Source: CAD feature listing. Evaluate the final solid. Frame: model axes, mm. Face numbers are marked on the shaded views. A direction names the side the tool comes from. Give positions to 0.01 mm unless a question says otherwise; leave off trailing zeros. Order: outer loops, then holes, each group sorted by start corner. A loop starts at its lowest first (then second) coordinate and runs counter-clockwise, first axis right, second up. Notation, with made-up numbers: (-23, 73.25) -> (-18, 73.25) arc R14 cw to (-18, 99.25) -> close; hole circle Ø11 at (-29, 5.5). An arc over 180 degrees is marked (long way). Answer in a Markdown table with one row per item.
```python
from build123d import *

# Parameters (mm, degrees)
SKETCH1_R           = 2
BOSS_EXTRUDE1_DEPTH = 3
SKETCH2_R           = 7
BOSS_EXTRUDE2_DEPTH = 9.35
SKETCH3_R           = 7.5
BOSS_EXTRUDE3_DEPTH = 0.5
SKETCH4_W           = 3
SKETCH4_H           = 9
BOSS_EXTRUDE4_DEPTH = 24.5
SKETCH5_R           = 6
BOSS_EXTRUDE5_DEPTH = 9.5
SKETCH8_R           = 5.5
BOSS_EXTRUDE6_DEPTH = 1.65
SKETCH9_R           = 7
BOSS_EXTRUDE7_DEPTH = 2
SKETCH10_R          = 4.5
CUT_EXTRUDE1_DEPTH  = 25
CUT_EXTRUDE2_DEPTH  = 3


with BuildPart() as part:
    # Sketch1 → Boss-Extrude1 (new body)
    with BuildSketch(Plane.XY):
        with BuildLine():
            ThreePointArc((-3.999511648, -14.062500079), (-8.7e-08, -16.5), (3.999511568, -14.062500234))
            Line((3.999511568, -14.062500234), (8.887803753, -4.583333333))
            ThreePointArc((8.887803753, -4.583333333), (10, 0), (8.887803753, 4.583333333))
            Line((8.887803753, 4.583333333), (3.999511579, 14.062500214))
            ThreePointArc((3.999511579, 14.062500214), (-6.7e-08, 16.5), (-3.99951164, 14.062500095))
            Line((-3.99951164, 14.062500095), (-8.887803753, 4.583333333))
            ThreePointArc((-8.887803753, 4.583333333), (-10, 0), (-8.887803753, -4.583333333))
            Line((-8.887803753, -4.583333333), (-3.999511648, -14.062500079))
        make_face()
        with Locations((0, -12)):
            Circle(SKETCH1_R, mode=Mode.SUBTRACT)
        with Locations((0, 12)):
            Circle(SKETCH1_R, mode=Mode.SUBTRACT)
    extrude(amount=BOSS_EXTRUDE1_DEPTH)

    # Sketch2 → Boss-Extrude2 (add)
    with BuildSketch(Plane.XY.offset(3)):
        Circle(SKETCH2_R)
    extrude(amount=BOSS_EXTRUDE2_DEPTH)

    # Sketch3 → Boss-Extrude3 (add)
    with BuildSketch(Plane(origin=(0, 0, 0), x_dir=(-1, 0, 0), z_dir=(0, 0, -1))):
        with Locations(Location((0, 0, 0), (0, 0, 180))):
            Circle(SKETCH3_R)
    extrude(amount=BOSS_EXTRUDE3_DEPTH)

    # Sketch4 → Boss-Extrude4 (add)
    with BuildSketch(Plane(origin=(0, 0, -0.5), x_dir=(-1, 0, 0), z_dir=(0, 0, -1))):
        Rectangle(SKETCH4_W, SKETCH4_H)
    extrude(amount=BOSS_EXTRUDE4_DEPTH)

    # Sketch5 → Boss-Extrude5 (add)
    with BuildSketch(Plane(origin=(0, 0, -0.5), x_dir=(-1, 0, 0), z_dir=(0, 0, -1))):
        Circle(SKETCH5_R)
    extrude(amount=BOSS_EXTRUDE5_DEPTH)

    # Sketch8 → Boss-Extrude6 (add)
    with BuildSketch(Plane.XY.offset(12.35)):
        Circle(SKETCH8_R)
    extrude(amount=BOSS_EXTRUDE6_DEPTH)

    # Sketch9 → Boss-Extrude7 (add)
    with BuildSketch(Plane.XY.offset(14)):
        Circle(SKETCH9_R)
    extrude(amount=BOSS_EXTRUDE7_DEPTH)

    # Sketch10 → Cut-Extrude1 (cut)
    with BuildSketch(Plane.XY.offset(16)):
        Circle(SKETCH10_R)
    extrude(amount=-CUT_EXTRUDE1_DEPTH, mode=Mode.SUBTRACT)

    # Sketch15 → Cut-Extrude2 (cut)
    with BuildSketch(Plane(origin=(1.5, 0, 0), x_dir=(0, 0, -1), z_dir=(1, 0, 0))):
        with BuildLine():
            Line((20, -2), (18, -2))
            ThreePointArc((18, -2), (16, 0), (18, 2))
            Line((18, 2), (20, 2))
            ThreePointArc((20, 2), (22, 0), (20, -2))
        make_face()
    extrude(amount=-CUT_EXTRUDE2_DEPTH, mode=Mode.SUBTRACT)


solid = part.part
```
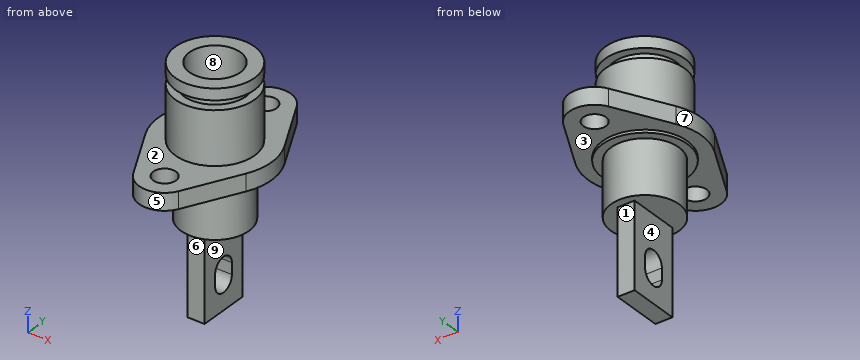
(1) Section query C-C (x = 0). Give the number of separate pieces and of enclosed holes in the cut face, plus the area to 3 significant figures.
A:
| item | result |
|---|---|
| separate pieces | 3 |
| enclosed holes | 1 |
| area | 263 mm^2 |
(2) Ray query, probe 1 along Y at (x, z) = (0, 0.75); probe 2 along Z at (x, y) = (6, 1); probe 3 along Y at (x, z) = (0, 6.5). Return the intervals inside material, ascending.
A:
| item | result |
|---|---|
| probe 1 | y = -16.5 to -14, -10 to -4.5, 4.5 to 10, 14 to 16.5 |
| probe 2 | z = -0.5 to 12.35, 14 to 16 |
| probe 3 | y = -7 to -4.5, 4.5 to 7 |
(3) Access query for the marked faces 1, 2, 3, 4 and 5. Directions: +Z, -Z, +X, -X, +Y, -Y. A direction counts if a zero-diameter tool reaches every point of the face in a straight line with its end or side. Return the directions, or none.
A:
| item | result |
|---|---|
| face 1 | -Z, +X, -X, +Y |
| face 2 | +Z |
| face 3 | -Z |
| face 4 | -Z, -X, +Y, -Y |
| face 5 | +Z, -Z, -Y |
(4) First-contact query: pin 1 Ø1.6 at (x, z) = (-0.5, -19) entering from -Y; pin 2 Ø10 at (y, z) = (-8.5, -1) entering from -X; pin 3 Ø1 at (x, y) = (-1.5, -8) entering from -Z; pin 4 Ø3.5 at (x, y) = (0, -12) entering from -Z. Flat tips, straight axial feed; report the tip coordinate or a pass-through.
A:
| item | result |
|---|---|
| pin 1 | stops at y = -4.5 |
| pin 2 | stops at x = -9.33 |
| pin 3 | stops at z = 0 |
| pin 4 | passes through |
(5) Pull-direction query (Y, two-part tool) for the marked faces 6, 7, 8 and 9; classes: +Y half, -Y half, draft (parallel to the pull), parting line (faces both ways), or undercut.
A:
| item | result |
|---|---|
| face 6 | -Y half |
| face 7 | parting line |
| face 8 | undercut |
| face 9 | draft |
(6) Section query A-A (z = -19). Return the cut outline in (x, y).
A:
| item | result |
|---|---|
| outline | (-1.5, -4.5) -> (1.5, -4.5) -> (1.5, -2) -> (-1.5, -2) -> close; (-1.5, 2) -> (1.5, 2) -> (1.5, 4.5) -> (-1.5, 4.5) -> close |
(7) Section query B-B (z = 1). Return the cut outline in (x, y).
A:
| item | result |
|---|---|
| outline | (-8.89, -4.58) -> (-4, -14.06) arc R4.5 ccw to (4, -14.06) -> (8.89, -4.58) arc R10 ccw to (8.89, 4.58) -> (4, 14.06) arc R4.5 ccw to (-4, 14.06) -> (-8.89, 4.58) arc R10 ccw to start; hole circle Ø9 at (0, 0); hole circle Ø4 at (0, -12); hole circle Ø4 at (0, 12) |
(8) Section query D-D (y = -12). Return the cut outline in (x, z).
A:
| item | result |
|---|---|
| outline | (-5.06, 0) -> (-2, 0) -> (-2, 3) -> (-5.06, 3) -> close; (2, 0) -> (5.06, 0) -> (5.06, 3) -> (2, 3) -> close |
